Check sheet for the modelled part. Datum: model origin and axes. Units: mm. A direction names the side the tool comes from. Round coordinates to 2 decimals unless told otherwise and drop trailing zeros. Write each loop counter-clockwise with the first axis right and the second up, starting at its lowest first coordinate (ties: lowest second). Pieces come first, ordered by that corner, then holes. Notation, with made-up numbers: (19, 10.25) - (46, 10.25) arc R12 ccw to (46, 23.25) - close; hole circle Ø8 at (88.25, 71.25). An arc over 180 degrees is marked (long way). Use one line per item in the form item = value. Start each with the question number.
1) Draft check along Y on faces 1 (the face through (-0.37, -9.16, 7.64)), 2 (the face through (0, -5, 8.65)), 3 (the face through (0, 10, 0)), 4 (the face through (0, 2, -8)). Enter one of: +Y half, -Y half, draft (parallel to the pull), parting line (faces both ways), or undercut.
2) Gauge pin test, flat ends, axial feed: P1, Ø0.9, axis at x = -2, z = -8, coming from the +Y side; P2, Ø1, axis at x = 6.5, z = -2.5, coming from the +Y side; P3, Ø5, axis at x = -6, z = -6.5, coming from the +Y side; P4, Ø2, axis at x = 0, y = -7.5, coming from the +Z side. Record the tip position at first contact, or that the pin passes through.
3) Section check A-A (x = 0). Record the boundary of the cut face in (y, z), then the cut area to 3 significant figures.
4) Set-up check for faces 5 (the face through (0, 3, -7.5)), 6 (the face through (-6.65, -7, 0)), 7 (the face through (0, -5, -8.65)), 8 (the face through (0, 2, 0)): record each of +Z, -Z, +X, -X, +Y, -Y from which the full face is reachable in a straight line by a thin tool's end or side.
5) Section check B-B (y = -7.5). Record the boundary of the cut face in (x, z).
6) Section check C-C (y = -12). Record the boundary of the cut face in (x, z).
7) Section check D-D (z = 0). Record the boundary of the cut face in (x, y).
8) Scan line: probe 1 along X at (y, z) = (-6, 3). Record every from-to range of solid material in increasing order.
from build123d import *

# Parameters (mm, degrees)
CROQUIS3_W                   = 17.3
CROQUIS3_H                   = 17.3
CROQUIS3_W_2                 = 13.3
CROQUIS3_H_2                 = 13.3
SALIENTE_EXTRUIR1_DEPTH      = 15
CROQUIS3_2_W                 = 17.3
CROQUIS3_2_H                 = 17.3
CROQUIS3_2_W_2               = 13.3
CROQUIS3_2_H_2               = 13.3
SALIENTE_EXTRUIR2_DEPTH      = 2
CORTAR_EXTRUIR1_DEPTH        = 20.3557485
CORTAR_EXTRUIR1_DEPTH_BACK   = 20.3557485
CROQUIS5_R                   = 1.7
SALIENTE_EXTRUIR4_DEPTH      = 8.65
SALIENTE_EXTRUIR4_DEPTH_BACK = 8.65
VACIADO1_START               = -6.65
VACIADO1_DEPTH               = 13.3


# Read off the part's stored shape, not the designer's step: Vaciado1
with BuildPart() as part:
    # Croquis3 → Saliente-Extruir1 (new body)
    with BuildSketch(Plane(origin=(0, 0, 0), x_dir=(1, 0, 0), z_dir=(0, 1, 0))):
        Rectangle(CROQUIS3_W, CROQUIS3_H)
        Rectangle(CROQUIS3_W_2, CROQUIS3_H_2, mode=Mode.SUBTRACT)
    extrude(amount=-SALIENTE_EXTRUIR1_DEPTH)

    # Croquis3<2> → Saliente-Extruir2 (add)
    # profile 1 of 2: a face of its own
    with BuildSketch(Plane(origin=(0, 0, 0), x_dir=(1, 0, 0), z_dir=(0, 1, 0))):
        Rectangle(CROQUIS3_2_W, CROQUIS3_2_H)
        Rectangle(CROQUIS3_2_W_2, CROQUIS3_2_H_2, mode=Mode.SUBTRACT)
    # profile 2 of 2: a face of its own
    with BuildSketch(Plane(origin=(0, 0, 0), x_dir=(1, 0, 0), z_dir=(0, 1, 0))):
        Rectangle(CROQUIS3_2_W_2, CROQUIS3_2_H_2)
    extrude(amount=SALIENTE_EXTRUIR2_DEPTH)

    # Croquis5 → Cortar-Extruir1 (cut, two sides: drawn at the far end of the back side and taken through both)
    with BuildSketch(Plane.XY.offset(-CORTAR_EXTRUIR1_DEPTH_BACK)):
        with Locations((0, -7.5)):
            Circle(CROQUIS5_R)
    extrude(amount=CORTAR_EXTRUIR1_DEPTH + CORTAR_EXTRUIR1_DEPTH_BACK, mode=Mode.SUBTRACT)

    # Croquis7 → Saliente-Extruir4 (add, two sides: drawn at the far end of the back side and taken through both)
    with BuildSketch(Plane(origin=(0, 0, 0), x_dir=(0, 0, -1), z_dir=(1, 0, 0)).offset(-SALIENTE_EXTRUIR4_DEPTH_BACK)):
        with BuildLine():
            Line((-7.5, 4.5), (-7.5, 2))
            Line((-7.5, 2), (7.5, 2))
            Line((7.5, 2), (7.5, 4.5))
            ThreePointArc((7.5, 4.5), (0, 12), (-7.5, 4.5))
        make_face()
    extrude(amount=SALIENTE_EXTRUIR4_DEPTH + SALIENTE_EXTRUIR4_DEPTH_BACK)

    # Vaciado1 outline → Vaciado1 (cut)
    with BuildSketch(Plane.YZ.offset(VACIADO1_START)):
        with BuildLine():
            Line((2, 5.5), (2, -5.5))
            Line((2, -5.5), (4.5, -5.5))
            ThreePointArc((4.5, -5.5), (10, 0), (4.5, 5.5))
            Line((4.5, 5.5), (2, 5.5))
        make_face()
    extrude(amount=VACIADO1_DEPTH, mode=Mode.SUBTRACT)


solid = part.part
Results are:
q1.face_1 = undercut
q1.face_2 = draft
q1.face_3 = undercut
q1.face_4 = +Y half
q2.P1 = 2
q2.P2 = 11.73
q2.P3 = 10.84
q2.P4 = through
q3.outline = (-15, -8.65) - (-9.2, -8.65) - (-9.2, -6.65) - (-15, -6.65) - close; (-15, 6.65) - (-9.2, 6.65) - (-9.2, 8.65) - (-15, 8.65) - close; (-5.8, -8.65) - (2, -8.65) - (2, -7.5) - (4.5, -7.5) arc R7.5 ccw to (4.5, 7.5) - (2, 7.5) - (2, 8.65) - (-5.8, 8.65) - (-5.8, 6.65) - (0, 6.65) - (0, -6.65) - (-5.8, -6.65) - close; hole (2, -5.5) - (4.5, -5.5) arc R5.5 ccw to (4.5, 5.5) - (2, 5.5) - close
q3.area = 132 mm²
q4.face_5 = -Z, +X, -X, +Y
q4.face_6 = -Y
q4.face_7 = -Z, +X, -X, +Y, -Y
q4.face_8 = none
q5.outline = (-8.65, -8.65) - (-1.7, -8.65) - (-1.7, -6.65) - (-6.65, -6.65) - (-6.65, 6.65) - (-1.7, 6.65) - (-1.7, 8.65) - (-8.65, 8.65) - close; (1.7, -8.65) - (8.65, -8.65) - (8.65, 8.65) - (1.7, 8.65) - (1.7, 6.65) - (6.65, 6.65) - (6.65, -6.65) - (1.7, -6.65) - close
q6.outline = (-8.65, -8.65) - (8.65, -8.65) - (8.65, 8.65) - (-8.65, 8.65) - close; hole (-6.65, -6.65) - (6.65, -6.65) - (6.65, 6.65) - (-6.65, 6.65) - close
q7.outline = (-8.65, -15) - (-6.65, -15) - (-6.65, 0) - (6.65, 0) - (6.65, -15) - (8.65, -15) - (8.65, 12) - (-8.65, 12) - close; hole (-6.65, 2) - (6.65, 2) - (6.65, 10) - (-6.65, 10) - close
q8.probe_1 = -8.65 to -6.65, 6.65 to 8.65
